Design review of the part built by this model. Coordinates are the model's own, in mm. A direction names the side the tool comes from. Give positions to 0.01 mm unless a question says otherwise; leave off trailing zeros. Loops run counter-clockwise (first coordinate to the right, second up) from the corner with the lowest first, then second, coordinate; pieces in that order, holes last. Notation, with made-up numbers: (-19, 78) - (16, 78) arc R20 cw to (16, 94) - close; hole circle Ø11 at (62.5, -26). An arc over 180 degrees is marked (long way). Write each question's results on one line, items separated by ' | '.
```python
from build123d import *

# Parameters (mm, degrees)
F0_W           = 6.5
F0_H           = 5
F0_W_2         = 10
F0_H_2         = 9
F1_DEPTH       = 3
F2_D           = 2.4
F2_DEPTH       = 3
F2_CBORE_D     = 4
F2_CBORE_DEPTH = 1
F2_TIP         = 0.7210327428
F3_R           = 1


# Not quite as in the source:
# - a feature names something its author has since deleted; it is built from what else it names


with BuildPart() as f1:
    # F0 (on Front) → F1 (new body)
    with BuildSketch(Plane.XZ):
        with Locations((8.25, -8.3)):
            Rectangle(F0_W, F0_H)
        with Locations((0, -8.3)):
            Rectangle(F0_W_2, F0_H)
        with Locations((-8.25, -8.3)):
            Rectangle(F0_W, F0_H)
        Polygon((5, -5.8), (11.5, -5.8), (11.5, 10.8), (-11.5, 10.8), (-11.5, -5.8), (-5, -5.8), align=None)
        with Locations((0, 2.5)):
            Rectangle(F0_W_2, F0_H_2, mode=Mode.SUBTRACT)
    extrude(amount=F1_DEPTH)

    # F2
    with Locations(Plane(origin=(0, 0, 0), x_dir=(1, 0, 0), z_dir=(0, 1, 0))):
        with Locations((7.5, 8.3), (-7.5, 8.3)):
            CounterBoreHole(F2_D / 2, F2_CBORE_D / 2, F2_CBORE_DEPTH, depth=F2_DEPTH)
            with Locations((0, 0, -(F2_DEPTH + F2_TIP / 2))):  # 118° drill point
                Cone(0, F2_D / 2, F2_TIP, mode=Mode.SUBTRACT)

    # F3
    f3_edges = [f1.edges().sort_by_distance(p)[0] for p in [
        (-11.5, 0, 0),
        (0, 0, 10.8),
        (11.5, -1.5, 10.8),
        (-11.5, -1.5, 10.8),
        (11.5, 0, 0),
        (-5, 0, 2.5),
        (0, 0, 7),
        (5, 0, 2.5),
        (0, 0, -2),
    ]]
    fillet(f3_edges, radius=F3_R)


solid = f1.part
```
Item 1: Draft analysis for pull direction X (two halves, no side actions). For faces 1 (the face through (-11.5, -2, 0)), 2 (the face through (-0.2, -3, -2.2)), 3 (the face through (-6.616, -2.014, -9.111)), state which applies: +X half, -X half, draft (parallel to the pull), parting line (faces both ways), or undercut.
Output values:
face 1: -X half | face 2: draft | face 3: undercut
Item 2: Wall thickness on probe 1 along X at (y, z) = (-1.45, -8.3); probe 2 along X at (y, z) = (-1.4, 5.75); probe 3 along Z at (x, y) = (7.5, -2.45): over which ranges is each line inside the solid? List them lowest first.
Output values:
probe 1: x = -11.5 to -8.7, -6.3 to 6.3, 8.7 to 11.5 | probe 2: x = -11.5 to -5, 5 to 11.5 | probe 3: z = -10.8 to -9.5, -7.1 to 10.8
Item 3: We need section D-D on z = 4.25. Give the boundary of the cut face in (x, y), then the cut area to 3 significant figures.
Output values:
outline: (-11.5, -3) - (-5, -3) - (-5, -1) arc R1 ccw to (-6, 0) - (-10.5, 0) arc R1 ccw to (-11.5, -1) - close; (5, -3) - (11.5, -3) - (11.5, -1) arc R1 ccw to (10.5, 0) - (6, 0) arc R1 ccw to (5, -1) - close | area: 38.1 mm²
Item 4: We need section C-C on y = -1.7. Give the boundary of the cut face in (x, z).
Output values:
outline: (-11.5, -10.8) - (11.5, -10.8) - (11.5, 9.8) arc R1 ccw to (10.5, 10.8) - (-10.5, 10.8) arc R1 ccw to (-11.5, 9.8) - close; hole circle Ø2.4 at (-7.5, -8.3); hole (-5, -2) - (5, -2) - (5, 7) - (-5, 7) - close; hole circle Ø2.4 at (7.5, -8.3)
Item 5: Clearance check with flat-ended pins moving along their axes: P1, Ø2.5, axis at x = 7.5, z = -8.3, coming from the -Y side; P2, Ø1.2, axis at x = -7.5, z = -9, coming from the +Y side. State where each tip first meets the part, or that it passes through.
Output values:
P1: stops at y = -3 | P2: stops at y = -1
Item 6: Tool access review of faces 4 (the face through (-5.285, -0.301, 2.577)), 5 (the face through (5, -2, 2)), 6 (the face through (11.215, -0.301, -0.356)): name each direction out of +Z, -Z, +X, -X, +Y, -Y from which nothing blocks a thin tool from reaching the whole face with its end or side.
Output values:
face 4: +Y | face 5: +Y, -Y | face 6: +Z, -Z, +X, +Y
Item 7: We need section A-A on x = -7.5. Give the boundary of the cut face in (y, z).
Output values:
outline: (-3, -10.8) - (0, -10.8) - (0, -10.3) - (-1, -10.3) - (-1, -9.5) - (-3, -9.5) - close; (-3, -7.1) - (-1, -7.1) - (-1, -6.3) - (0, -6.3) - (0, 9.8) arc R1 ccw to (-1, 10.8) - (-3, 10.8) - close
Item 8: We need section B-B on z = -8.3. Give the boundary of the cut face in (x, y).
Output values:
outline: (-11.5, -3) - (-8.7, -3) - (-8.7, -1) - (-9.5, -1) - (-9.5, 0) - (-10.5, 0) arc R1 ccw to (-11.5, -1) - close; (-6.3, -3) - (6.3, -3) - (6.3, -1) - (5.5, -1) - (5.5, 0) - (-5.5, 0) - (-5.5, -1) - (-6.3, -1) - close; (8.7, -3) - (11.5, -3) - (11.5, -1) arc R1 ccw to (10.5, 0) - (9.5, 0) - (9.5, -1) - (8.7, -1) - close
